Answer from the drawing. Dimensions are ordinates in mm from the lowest x, y and z of the part. Round coordinates to 2 decimals unless told otherwise and drop trailing zeros. Write each loop counter-clockwise with the first axis right and the second up, starting at its lowest first coordinate (ties: lowest second). Pieces come first, ordered by that corner, then holes. Notation, with made-up numbers: (78, 5) -> (121, 5) arc R11 ccw to (121, 22) -> close; hole circle Ø5 at (-34, 4). An arc over 180 degrees is marked (long way). Return JSON: item names as keys, results as strings. Group by question number.
(1) A cutting plane is placed at A-A on z = 33. Give the vertices of the cut face in (x, y).
(2) A cutting plane is placed at B-B on z = 9. Give the vertices of the cut face in (x, y).
(3) Straight lines are drawn through the part: line 1 (Z direction, x = 3.25, y = 6.25); line 2 (X direction, y = 3.75, z = 94); line 3 (Y direction, x = 0.75, z = 67) (1 decimal). For each, find the intervals that lie inside material, in ascending order.
(4) Given pin 1 (1 mm diameter, centred on x = 3, y = 1.5, fed in from -Z); pin 2 (1.5 mm diameter, centred on x = 4.5, y = 3.5, fed in from +Z); pin 3 (3 mm diameter, centred on x = 3.5, y = 4.04, fed in from +Z), each flat-ended and moving along its own axis, determine where each tip first touches the part or whether it passes through.
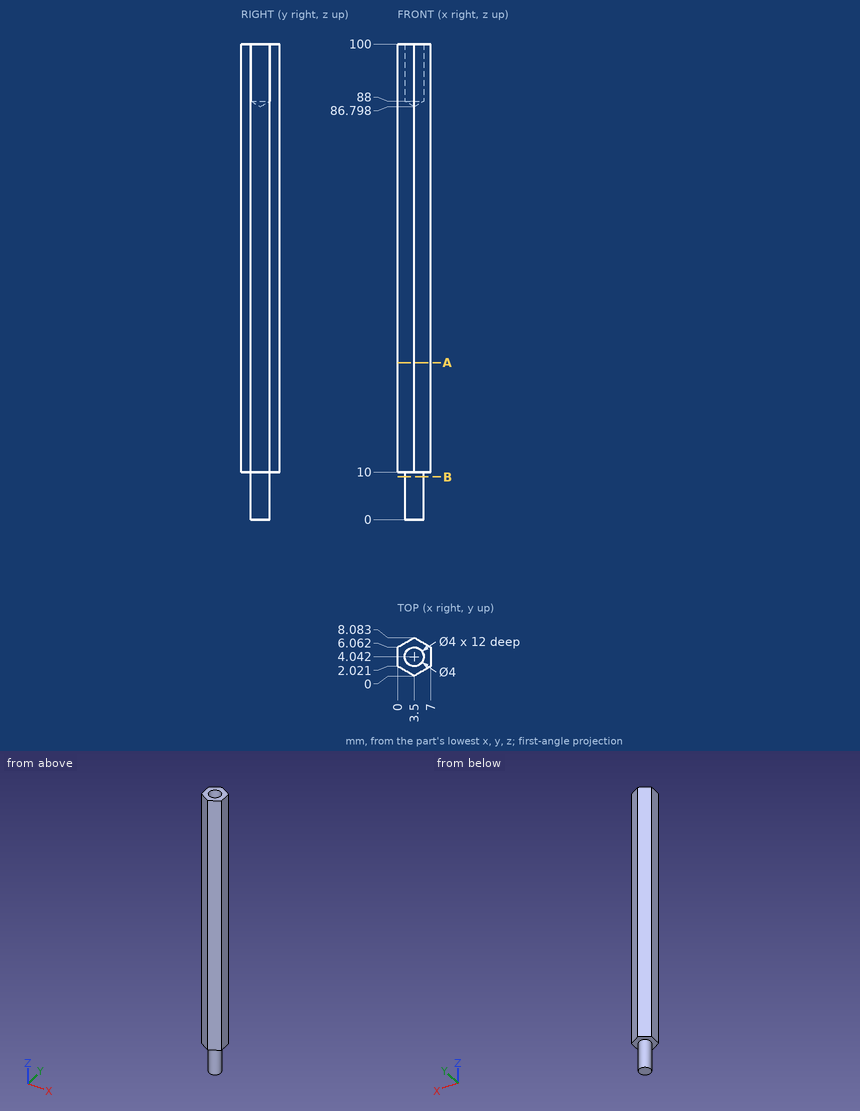
Checks:
{
 "1": {"outline": "(0, 2.02) -> (3.5, 0) -> (7, 2.02) -> (7, 6.06) -> (3.5, 8.08) -> (0, 6.06) -> close"},
 "2": {"outline": "circle Ø4 at (3.5, 4.04)"},
 "3": {"line 1": "z = 10 to 100", "line 2": "x = 0 to 1.52, 5.48 to 7", "line 3": "y = 1.6 to 6.5"},
 "4": {"pin 1": "stops at z = 10", "pin 2": "stops at z = 87.93", "pin 3": "stops at z = 87.7"}
}
